Here's how the part is built. I have some questions about the finished solid (model axes, mm). A direction names the side the tool comes from. Give positions to 0.01 mm unless a question says otherwise; leave off trailing zeros. Loops run counter-clockwise (first coordinate to the right, second up) from the corner with the lowest first, then second, coordinate; pieces in that order, holes last. Notation, with made-up numbers: (-7.75, 11) -> (43.25, 11) arc R28 ccw to (43.25, 33) -> close; hole circle Ø2 at (71, -29.75). An arc over 180 degrees is marked (long way). Answer in a Markdown table with one row per item. Add a question column.
Item 1: If we section it at B-B (z = 0): Give the number of separate pieces and of enclosed holes in the cut face, then the cut area to 3 significant figures.
Item 2: If we section it at C-C (y = 20): Write out the boundary of the cut face in (x, z), then the cut area to 3 significant figures.
Item 3: For P1, Ø1.5, axis at x = -3.5, z = -1.5, coming from the +Y side; P2, Ø3.5, axis at x = -15, y = 26.5, coming from the +Z side; P3, Ø1.5, axis at y = 1, z = -11, coming from the +X side; P4, Ø4, axis at x = 17.5, z = -2.5, coming from the +Y side, each with a flat end and sliding along its axis, tell me the tip position at first contact or that it passes through.
Item 4: We'd pull the mould along X, two halves only. Please class faces 6 (the face through (-39, 0, 0)), 7 (the face through (41, -2, 0)), 8 (the face through (-11.5, 16, 9)): released by +X, released by -X, zero draft, split by the parting line, or undercut.
Item 5: If we section it at D-D (z = 5): Write out the boundary of the cut face in (x, y).
Item 6: Which directions (+Z, -Z, +X, -X, +Y, -Y) give clear straight access to the entire face, cutting with the end or side of a thin tool? Please do faces 1 (the face through (18.824, 12.325, 8.961)), 2 (the face through (0, 9, -9)), 3 (the face through (19, 25, 0)), 4 (the face through (-16, 27, 2.75)), 5 (the face through (-41, -2, 0)).
Item 7: If we section it at A-A (x = 0): Write out the boundary of the cut face in (y, z).
Item 8: If I drill on line 1 (Z direction, x = 1, y = 5); line 2 (Y direction, x = 33, z = -6.5); line 3 (Y direction, x = 2, z = 3), over which ranges is the centre line in solid material (lowest first)?
```python
from build123d import *

# Parameters (mm, degrees)
BOSS_EXTRUDE1_DEPTH     = 4
BOSS_EXTRUDE2_DEPTH     = 30
BOSS_EXTRUDE3_DEPTH     = 11.5
CUT_EXTRUDE1_DEPTH      = 57.160484328
CUT_EXTRUDE1_DEPTH_BACK = 57.160484328
SKETCH4_3_W             = 3
SKETCH4_3_H             = 3
BOSS_EXTRUDE4_DEPTH     = 2.75
SKETCH5_W               = 21
SKETCH5_H               = 18
CUT_EXTRUDE3_DEPTH      = 27
M4_CLEARANCE_HOLE1_D    = 4.5


with BuildPart() as part:
    # Sketch2 → Boss-Extrude1 (new body)
    with BuildSketch(Plane(origin=(0, 0, 0), x_dir=(1, 0, 0), z_dir=(0, 1, 0))):
        with BuildLine():
            Line((-43, 15), (43, 15))
            ThreePointArc((43, 15), (46.535533906, 13.535533906), (48, 10))
            Line((48, 10), (48, -10))
            ThreePointArc((48, -10), (46.535533906, -13.535533906), (43, -15))
            Line((43, -15), (-43, -15))
            ThreePointArc((-43, -15), (-46.535533906, -13.535533906), (-48, -10))
            Line((-48, -10), (-48, 10))
            ThreePointArc((-48, 10), (-46.535533906, 13.535533906), (-43, 15))
        make_face()
        with BuildLine():
            Line((-46, -7.5), (-46, 7.5))
            ThreePointArc((-46, 7.5), (-43.5, 10), (-41, 7.5))
            Line((-41, 7.5), (-41, -7.5))
            ThreePointArc((-41, -7.5), (-43.5, -10), (-46, -7.5))
        make_face(mode=Mode.SUBTRACT)
        with BuildLine():
            Line((46, -7.5), (46, 7.5))
            ThreePointArc((46, 7.5), (43.5, 10), (41, 7.5))
            Line((41, 7.5), (41, -7.5))
            ThreePointArc((41, -7.5), (43.5, -10), (46, -7.5))
        make_face(mode=Mode.SUBTRACT)
    extrude(amount=-BOSS_EXTRUDE1_DEPTH)

    # Sketch3 → Boss-Extrude2 (add, symmetric)
    with BuildSketch(Plane(origin=(0, 0, 0), x_dir=(0, 0, -1), z_dir=(1, 0, 0))):
        Polygon((-15, 0), (-2.75, 25), (2.75, 25), (15, 0), align=None)
    extrude(amount=BOSS_EXTRUDE2_DEPTH, both=True)

    # Sketch3<3> → Boss-Extrude3 (add, symmetric)
    with BuildSketch(Plane(origin=(0, 0, 0), x_dir=(0, 0, -1), z_dir=(1, 0, 0))):
        Polygon((-10, 25), (-15, 0), (-2.75, 25), align=None)
        Polygon((2.75, 25), (15, 0), (10, 25), align=None)
    extrude(amount=BOSS_EXTRUDE3_DEPTH, both=True)

    # Sketch4 → Cut-Extrude1 (cut, two sides: drawn at the far end of the back side and taken through both)
    with BuildSketch(Plane.XY.offset(-CUT_EXTRUDE1_DEPTH_BACK)):
        Polygon((21, 25), (30, 0), (30, 25), align=None)
        Polygon((-30, 25), (-30, 0), (-21, 25), align=None)
    extrude(amount=CUT_EXTRUDE1_DEPTH + CUT_EXTRUDE1_DEPTH_BACK, mode=Mode.SUBTRACT)

    # Sketch4<3> → Boss-Extrude4 (add, symmetric)
    with BuildSketch(Plane.XY):
        with Locations((15.5, 26.5)):
            Rectangle(SKETCH4_3_W, SKETCH4_3_H)
        with Locations((-15.5, 26.5)):
            Rectangle(SKETCH4_3_W, SKETCH4_3_H)
    extrude(amount=BOSS_EXTRUDE4_DEPTH, both=True)

    # Sketch5 → Cut-Extrude3 (cut)
    with BuildSketch(Plane.XZ.offset(4)):
        Rectangle(SKETCH5_W, SKETCH5_H)
    extrude(amount=-CUT_EXTRUDE3_DEPTH, mode=Mode.SUBTRACT)

    # M4 Clearance Hole1 (through all)
    with Locations(Plane(origin=(0, 25, 0), x_dir=(1, 0, 0), z_dir=(0, 1, 0))):
        with Locations((0, 0)):
            Hole(M4_CLEARANCE_HOLE1_D / 2)


solid = part.part
```
Recorded:
| question | item | result |
|---|---|---|
| 1 | separate pieces | 4 |
| 1 | enclosed holes | 0 |
| 1 | area | 1,060 mm^2 |
| 2 | outline | (-22.8, -5.2) -> (-11.5, -5.2) -> (-11.5, -11) -> (11.5, -11) -> (11.5, -5.2) -> (22.8, -5.2) -> (22.8, 5.2) -> (11.5, 5.2) -> (11.5, 11) -> (-11.5, 11) -> (-11.5, 5.2) -> (-22.8, 5.2) -> close; hole (-10.5, -9) -> (10.5, -9) -> (10.5, 9) -> (-10.5, 9) -> close |
| 2 | area | 363 mm^2 |
| 3 | P1 | stops at y = 25 |
| 3 | P2 | stops at z = 2.87 |
| 3 | P3 | stops at x = 29.91 |
| 3 | P4 | stops at y = 28 |
| 4 | face 6 | zero draft |
| 4 | face 7 | undercut |
| 4 | face 8 | released by -X |
| 5 | outline | (-48, -4) -> (-46, -4) -> (-46, 0) -> (-48, 0) -> close; (-41, -4) -> (-10.5, -4) -> (-10.5, 23) -> (10.5, 23) -> (10.5, -4) -> (41, -4) -> (41, 0) -> (30, 0) -> (22.65, 20.41) -> (11.5, 20.41) -> (11.5, 25) -> (-11.5, 25) -> (-11.5, 20.41) -> (-22.65, 20.41) -> (-30, 0) -> (-41, 0) -> close; (46, -4) -> (48, -4) -> (48, 0) -> (46, 0) -> close |
| 6 | face 1 | +Z, +X, +Y |
| 6 | face 2 | -Y |
| 6 | face 3 | +Z, -Z, +X, +Y |
| 6 | face 4 | +Z, +X, -X, +Y |
| 6 | face 5 | +Y, -Y |
| 7 | outline | (-4, -15) -> (0, -15) -> (25, -10) -> (25, -2.25) -> (23, -2.25) -> (23, -9) -> (-4, -9) -> close; (-4, 9) -> (23, 9) -> (23, 2.25) -> (25, 2.25) -> (25, 10) -> (0, 15) -> (-4, 15) -> close |
| 8 | line 1 | z = -14 to -9, 9 to 14 |
| 8 | line 2 | y = -4 to 0 |
| 8 | line 3 | y = 23 to 25 |
